```python
from build123d import *

# Parameters (mm, degrees)
SKETCH_1_W      = 34.4
SKETCH_1_H      = 10
EXTRUDE_1_DEPTH = 0.5
EXTRUDE_2_DEPTH = 34.4


with BuildPart() as part:
    # Эскиз1 → Бобышка-Вытянуть1 (new body)
    with BuildSketch(Plane(origin=(0, 0, 0), x_dir=(1, 0, 0), z_dir=(0, 1, 0))):
        Rectangle(SKETCH_1_W, SKETCH_1_H)
    extrude(amount=EXTRUDE_1_DEPTH)

    # Эскиз2 → Бобышка-Вытянуть2 (add, through all)
    with BuildSketch(Plane.ZY.offset(17.2)):
        with BuildLine():
            ThreePointArc((5, 0.5), (0, 2.400988005), (-5, 0.5))
            Line((-5, 0.5), (-4.3, 0.5))
            ThreePointArc((-4.3, 0.5), (0, 1.9), (4.3, 0.5))
            Line((4.3, 0.5), (5, 0.5))
        make_face()
    extrude(amount=-EXTRUDE_2_DEPTH)


solid = part.part
```
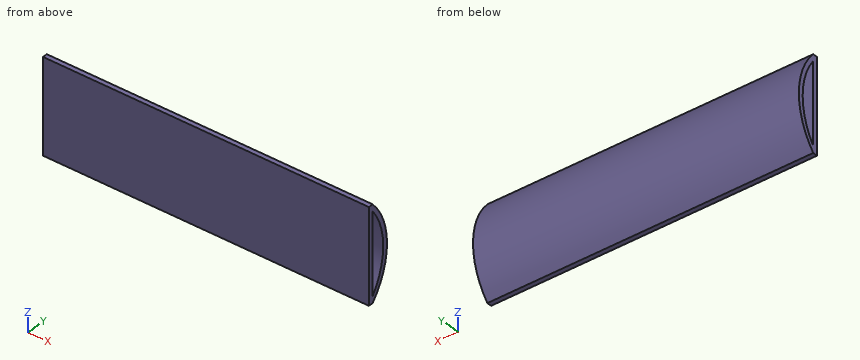
Work out the finished part from the listing and answer in its coordinate system (mm). Give positions to 0.01 mm unless a question says otherwise; leave off trailing zeros. Loops run counter-clockwise (first coordinate to the right, second up) from the corner with the lowest first, then second, coordinate; pieces in that order, holes last. Notation, with made-up numbers: (65, 77.25) -> (76, 77.25) arc R20 cw to (76, 99.25) -> close; hole circle Ø10 at (40.5, 66). An arc over 180 degrees is marked (long way). Use CSV: the item, a comma, the result in double quotes.
1. The part is cut by section A-A (y = 1.3). Write down the section's boundary in (x, z), then the cut area to 3 significant figures.
Found:
outline,"(-17.2, -3.92) -> (17.2, -3.92) -> (17.2, -2.9) -> (-17.2, -2.9) -> close; (-17.2, 2.9) -> (17.2, 2.9) -> (17.2, 3.92) -> (-17.2, 3.92) -> close"
area,"70.2 mm^2"
2. A flat-ended cylindrical pin translates along its axis: pin 1 Ø2.5 at (x, z) = (-5.5, 1) entering from +Y. Find the tip coordinate at first contact, or state that the pin passes through.
Found:
pin 1,"y = 2.4"
3. Straight lines are drawn through the part: line 1 (Y direction, x = 13, z = -0.25); line 2 (Y direction, x = -8, z = -3.25); line 3 (Z direction, x = -14.5, y = 1.3). For each, find the intervals that lie inside material, in ascending order.
Found:
line 1,"0 to 0.5, 1.9 to 2.4"
line 2,"0 to 0.5, 1.14 to 1.66"
line 3,"-3.92 to -2.9, 2.9 to 3.92"
4. The part is cut by section B-B (z = 3.5). Write down the section's boundary in (x, y).
Found:
outline,"(-17.2, 0) -> (17.2, 0) -> (17.2, 0.5) -> (-17.2, 0.5) -> close; (-17.2, 1.01) -> (17.2, 1.01) -> (17.2, 1.54) -> (-17.2, 1.54) -> close"
5. The part is cut by section C-C (x = -0.5). Write down the section's boundary in (y, z).
Found:
outline,"(0, -5) -> (0.5, -5) arc R7.53 ccw to (0.5, 5) -> (0, 5) -> close; hole (0.5, -4.3) arc R7.3 ccw to (0.5, 4.3) -> close"
